```python
from build123d import *

# Parameters (mm, degrees)
SKETCH1_W           = 54.737
SKETCH1_H           = 9.525
BOSS_EXTRUDE1_DEPTH = 1.5875
FILLET1_R           = 3.81
SKETCH2_R           = 1.4224
CUT_EXTRUDE1_DEPTH  = 2.5875


with BuildPart() as part:
    # Sketch1 → Boss-Extrude1 (new body)
    with BuildSketch(Plane(origin=(0, 0, 0), x_dir=(1, 0, 0), z_dir=(0, 1, 0))):
        with Locations((27.3685, 4.7625)):
            Rectangle(SKETCH1_W, SKETCH1_H)
    extrude(amount=BOSS_EXTRUDE1_DEPTH)

    # Fillet1
    fillet1_edges = [part.edges().sort_by_distance(p)[0] for p in [
        (0, 0.79375, -9.525),
        (54.737, 0.79375, -9.525),
        (54.737, 0.79375, 0),
        (0, 0.79375, 0),
    ]]
    fillet(fillet1_edges, radius=FILLET1_R)

    # Sketch2 → Cut-Extrude1 (cut, through all)
    with BuildSketch(Plane(origin=(0, 1.5875, 0), x_dir=(1, 0, 0), z_dir=(0, 1, 0))):
        with Locations((4.2545, 4.7625)):
            Circle(SKETCH2_R)
        with Locations((50.4825, 4.7625)):
            Circle(SKETCH2_R)
    extrude(amount=-CUT_EXTRUDE1_DEPTH, mode=Mode.SUBTRACT)


solid = part.part
```
Check sheet for the modelled part. Datum: model origin and axes. Units: mm. Coordinates: 2 decimals unless noted, no trailing zeros. Loops run counter-clockwise (first coordinate to the right, second up) from the corner with the lowest first, then second, coordinate; pieces in that order, holes last.
1) Sectioned sample at D-D (z = -8.25). Record the boundary of the cut face in (x, y), and give its area (3 significant figures).
2) Material ranges on probe 1 along X at (y, z) = (1.3, -6); probe 2 along X at (y, z) = (0.25, -5.75); probe 3 along X at (y, z) = (1.05, -7.25), recorded low to high.
3) Release check for a two-part mould opening along Z. For faces 1 (the face through (0, 1, -5)), 2 (the face through (27, 1, 0)), 3 (the face through (49.06, 0.8, -4.83)) record: released by +Z, released by -Z, zero draft, split by the parting line, or undercut.
4) Sectioned sample at B-B (y = 0.4). Record the boundary of the cut face in (x, z) (1 decimal).
5) Sectioned sample at C-C (x = 50). Record the boundary of the cut face in (y, z) (1 decimal).
6) Sectioned sample at A-A (x = 4.5). Record the boundary of the cut face in (y, z) (1 decimal), and give its area (3 significant figures).
Check sheet entries:
1. outline: (0.97, 0) - (53.77, 0) - (53.77, 1.59) - (0.97, 1.59) - close
1. area: 83.8 mm2
2. probe 1: x = 0.01 to 3.55, 4.96 to 49.78, 51.18 to 54.73
2. probe 2: x = 0 to 3.23, 5.28 to 49.46, 51.51 to 54.74
2. probe 3: x = 0.32 to 54.41
3. face 1: zero draft
3. face 2: released by +Z
3. face 3: undercut
4. outline: (0, -5.7) arc R3.8 ccw to (3.8, -9.5) - (50.9, -9.5) arc R3.8 ccw to (54.7, -5.7) - (54.7, -3.8) arc R3.8 ccw to (50.9, 0) - (3.8, 0) arc R3.8 ccw to (0, -3.8) - close; hole circle Ø2.8 at (4.3, -4.8); hole circle Ø2.8 at (50.5, -4.8)
5. outline: (0, -9.5) - (1.6, -9.5) - (1.6, -6.1) - (0, -6.1) - close; (0, -3.4) - (1.6, -3.4) - (1.6, 0) - (0, 0) - close
6. outline: (0, -9.5) - (1.6, -9.5) - (1.6, -6.2) - (0, -6.2) - close; (0, -3.4) - (1.6, -3.4) - (1.6, 0) - (0, 0) - close
6. area: 10.7 mm2
